Here's how the part is built. I have some questions about the finished solid (model axes, mm). A direction names the side the tool comes from. Round coordinates to 2 decimals unless told otherwise and drop trailing zeros. Order: outer loops, then holes, each group sorted by start corner. A loop starts at its lowest first (then second) coordinate and runs counter-clockwise, first axis right, second up. Notation, with made-up numbers: M -17.5,88 L 40.5,88 A26 ccw 40.5,126 Z; hole C 32,-12 d9. An arc over 180 degrees is marked long. Write item = value, one per line. Start each with the question number.
Item 1: I want a section at D-D, the plane z = 50.5. List the corners of the cut face in (x, y) for me, plus the area to 3 significant figures.
Item 2: I want a section at C-C, the plane x = 120. List the corners of the cut face in (y, z) for me, plus the area to 3 significant figures.
Item 3: Please list where these lines run through material, in increasing order: L1, parallel to Y at x = 120, z = 28; L2, parallel to Y at x = 120, z = 47.5; L3, parallel to Z at x = 85.5, y = 35.
Item 4: For faces 1 (the face through (70, 77, 2)), 2 (the face through (155, 85, 45)), 3 (the face through (90, 15, 55)), 4 (the face through (111, 80, 55)), 5 (the face through (111, 90, 50)), which set-ups out of +Z, -Z, +X, -X, +Y, -Y let a thin tool reach every point of the face, with its end or its side?
Item 5: I want a section at A-A, the plane z = 32.5. List the corners of the cut face in (x, y) for me, plus the area to 3 significant figures.
Item 6: I want a section at B-B, the plane y = 62. List the corners of the cut face in (x, z) for me.
Item 7: I'm going to push flat-ended pins straight in: P1, Ø24, axis at y = 87.5, z = 55, coming from the -X side; P2, Ø4.5, axis at y = 92.5, z = 5.5, coming from the -X side; P3, Ø6, axis at x = 90, y = 19.5, coming from the +Z side; P4, Ø10, axis at x = 175, z = 36, coming from the -Y side. Where does each tip first touch, or does it pass through?
Item 8: We'd pull the mould along Y, two halves only. Please class faces 6 (the face through (90, 90, 2)), 7 (the face through (2.8, 50, 2.8)), 8 (the face through (90, 15, 30)): pulls with the +Y half, pulls with the -Y half, needs draft (parallel to the pull), parting line crosses it, or undercut.
```python
from build123d import *

# Parameters (mm, degrees)
SKICA1_W                 = 200
SKICA1_H                 = 100
P_IDAT_VYSUNUT_M1_DEPTH  = 20
P_IDAT_VYSUNUT_M2_DEPTH  = 50
SKICA7_R                 = 7.5
P_IDAT_VYSUNUT_M3_DEPTH  = 50
ODEBRAT_VYSUNUT_M3_DEPTH = 10
ZAOBLIT1_START           = 50
ZAOBLIT1_DEPTH           = 51
SKICA9_W                 = 40
SKICA9_H                 = 25
ODEBRAT_VYSUNUT_M4_DEPTH = 5
CHAMFER2_SIZE            = 5
FILLET2_DEPTH            = 50
CHAMFER3_SIZE            = 40
CHAMFER3_SIZE2           = 20
CHAMFER4_SIZE            = 20
SKETCH3_R                = 15
CUT_EXTRUDE2_DEPTH       = 60
SKETCH4_W                = 10
SKETCH4_H                = 20
CUT_EXTRUDE3_DEPTH       = 22
SKETCH5_W                = 20
SKETCH5_H                = 10
BOSS_EXTRUDE1_DEPTH      = 30


with BuildPart() as part:
    # Skica1 → Přidat vysunutím1 (new body)
    with BuildSketch(Plane.XY):
        with Locations((100, 50)):
            Rectangle(SKICA1_W, SKICA1_H)
    extrude(amount=P_IDAT_VYSUNUT_M1_DEPTH)

    # Skica2 → Přidat vysunutím2 (add)
    with BuildSketch(Plane.XY.offset(20)):
        Polygon((100, 0), (200, 0), (200, 100), (155, 100), (155, 70), (130, 70), (130, 100), (100, 100), align=None)
    extrude(amount=P_IDAT_VYSUNUT_M2_DEPTH)

    # Skica7 → Přidat vysunutím3 (add)
    with BuildSketch(Plane.XY.offset(20)):
        with Locations(Location((12, 80, 0), (0, 0, 180))):
            Circle(SKICA7_R)
    extrude(amount=P_IDAT_VYSUNUT_M3_DEPTH)

    # Skica8 → Odebrat vysunutím3 (cut, symmetric)
    with BuildSketch(Plane.ZY.offset(-50)):
        Polygon((0, 100), (0, 70), (15, 100), align=None)
    extrude(amount=ODEBRAT_VYSUNUT_M3_DEPTH, both=True, mode=Mode.SUBTRACT)

    # Zaoblit1: read off the stored shape, not the designer's step
    # Zaoblit1 outline → Zaoblit1 (cut)
    with BuildSketch(Plane(origin=(0, 0, 0), x_dir=(1, 0, 0), z_dir=(0, 1, 0)).offset(ZAOBLIT1_START)):
        with BuildLine():
            ThreePointArc((0, -10), (2.928932188, -2.928932188), (10, 0))
            Line((10, 0), (0, 0))
            Line((0, 0), (0, -10))
        make_face()
    extrude(amount=ZAOBLIT1_DEPTH, mode=Mode.SUBTRACT)

    # Skica9 → Odebrat vysunutím4 (cut)
    with BuildSketch(Plane(origin=(0, 0, 0), x_dir=(-1, 0, 0), z_dir=(0, 0, -1))):
        with Locations((-90, 77.5)):
            Rectangle(SKICA9_W, SKICA9_H)
    extrude(amount=-ODEBRAT_VYSUNUT_M4_DEPTH, mode=Mode.SUBTRACT)

    # Chamfer2
    chamfer2_edges = [part.edges().sort_by_distance(p)[0] for p in [
        (0, 25, 0),
    ]]
    chamfer(chamfer2_edges, length=CHAMFER2_SIZE)

    # Fillet2: read off the stored shape, not the designer's step
    # Fillet2 outline → Fillet2 (cut)
    with BuildSketch(Plane(origin=(0, 0, 0), x_dir=(1, 0, 0), z_dir=(0, 1, 0))):
        with BuildLine():
            Line((200, 0), (140, 0))
            ThreePointArc((140, 0), (182.426406871, -17.573593129), (200, -60))
            Line((200, -60), (200, 0))
        make_face()
    extrude(amount=FILLET2_DEPTH, mode=Mode.SUBTRACT)

    # Chamfer3
    chamfer3_edges = [part.edges().sort_by_distance(p)[0] for p in [
        (200, 75, 0),
    ]]
    chamfer3_side = [part.faces().sort_by_distance(p)[0] for p in [
        (93.302047782, 51.38225256, 0),
    ]]
    chamfer(chamfer3_edges, length=CHAMFER3_SIZE, length2=CHAMFER3_SIZE2, reference=chamfer3_side[0])

    # Chamfer4
    chamfer4_edges = [part.edges().sort_by_distance(p)[0] for p in [
        (200, 75, 20),
    ]]
    chamfer(chamfer4_edges, length=CHAMFER4_SIZE)

    # Sketch2 → Cut-Revolve4 (revolve, cut)
    with BuildSketch(Plane(origin=(0, 0, 0), x_dir=(-1, 0, 0), z_dir=(0, 0, -1))):
        with BuildLine():
            Line((-50, 35), (-50, 5))
            ThreePointArc((-50, 5), (-35, 20), (-50, 35))
        make_face()
    revolve(axis=Axis((50, 35, 0), (0, -1, 0)), mode=Mode.SUBTRACT)

    # Sketch3 → Cut-Extrude2 (cut)
    with BuildSketch(Plane(origin=(0, 0, 0), x_dir=(-1, 0, 0), z_dir=(0, 0, -1))):
        with Locations((-120, 20)):
            Circle(SKETCH3_R)
    extrude(amount=-CUT_EXTRUDE2_DEPTH, mode=Mode.SUBTRACT)

    # Sketch4 → Cut-Extrude3 (cut)
    with BuildSketch(Plane.ZY.offset(-100)):
        with Locations((50, 80)):
            Rectangle(SKETCH4_W, SKETCH4_H)
    extrude(amount=-CUT_EXTRUDE3_DEPTH, mode=Mode.SUBTRACT)

    # Sketch5 → Boss-Extrude1 (add)
    with BuildSketch(Plane.XZ):
        Polygon((80, 55), (100, 40), (100, 55), align=None)
        with Locations((90, 35)):
            Rectangle(SKETCH5_W, SKETCH5_H)
    extrude(amount=-BOSS_EXTRUDE1_DEPTH)


solid = part.part
```
Filled in:
q1.outline = C 12,80 d15; M 86,0 L 199.24,0 L 199.24,50 L 200,50 L 200,100 L 155,100 L 155,70 L 130,70 L 130,100 L 100,100 L 100,90 L 122,90 L 122,70 L 100,70 L 100,30 L 86,30 Z; hole C 120,20 d30
q1.area = 8,660 mm^2
q2.outline = M 0,0 L 5,0 L 5,60 L 35,60 L 35,0 L 100,0 L 100,70 L 0,70 Z; hole M 70,45 L 90,45 L 90,55 L 70,55 Z
q2.area = 5,000 mm^2
q3.L1 = 0 to 5, 35 to 100
q3.L2 = 0 to 5, 35 to 70, 90 to 100
q3.L3 = 0 to 20
q4.face_1 = -Z
q4.face_2 = +Z, +Y
q4.face_3 = +Z, -X, +Y, -Y
q4.face_4 = none
q4.face_5 = -X
q5.outline = C 12,80 d15; M 80,0 L 193.33,0 L 193.33,50 L 195.36,50 L 195.36,100 L 155,100 L 155,70 L 130,70 L 130,100 L 100,100 L 100,30 L 80,30 Z; hole C 120,20 d30
q5.area = 8,750 mm^2
q6.outline = M 0,10 A10 ccw 10,0 L 160,0 L 182.11,11.06 L 200,40 L 200,70 L 100,70 L 100,20 L 0,20 Z
q7.P1 = 4.5
q7.P2 = 0.26
q7.P3 = 55
q7.P4 = 0
q8.face_6 = undercut
q8.face_7 = pulls with the +Y half
q8.face_8 = needs draft
